The model under review builds one solid part; all positions refer to its coordinate system, in mm. A direction names the side the tool comes from. Give positions to 0.01 mm unless a question says otherwise; leave off trailing zeros. Write each loop counter-clockwise with the first axis right and the second up, starting at its lowest first coordinate (ties: lowest second). Pieces come first, ordered by that corner, then holes. Notation, with made-up numbers: (52.5, -27) -> (105.5, -27) arc R23 cw to (105.5, -19) -> close; hole circle Ø5 at (56.25, 46). An arc over 180 degrees is marked (long way). Use CSV: the item, a comma, the result in double quotes.
```python
from build123d import *

# Parameters (mm, degrees)
F1_DEPTH = 30
F2_R     = 0.5


with BuildPart() as f1:
    # F0 (on Front) → F1 (new body, symmetric)
    with BuildSketch(Plane.XZ):
        Polygon((-63.04628, 0), (0, 0), (0, 3), (-4.215537, 9.893654), (-3, 3), (-15, 3), (-22.38508, 44.88287), (-25.860448, 47.316349), (-18.04628, 3), (-63.04628, 3), align=None)
    extrude(amount=F1_DEPTH, both=True)

    # F2
    f2_edges = [f1.edges().sort_by_distance(p)[0] for p in [
        (-22.38508, 0, 44.88287),
        (-4.215537, 0, 9.893654),
        (-25.860448, 0, 47.316349),
    ]]
    fillet(f2_edges, radius=F2_R)


solid = f1.part
```
Q1. Consider section C-C (x = -19.5). Write out the cut boundary in (y, z).
Derived:
outline,"(-30, 0) -> (30, 0) -> (30, 3) -> (-30, 3) -> close; (-30, 11.24) -> (30, 11.24) -> (30, 28.52) -> (-30, 28.52) -> close"
Q2. Insertion check: pin 1 (22.5 mm diameter, centred on x = -45, y = 6.5, fed in from +Z); pin 2 (13 mm diameter, centred on x = -8.5, y = -9.5, fed in from +Z). Each pin has a flat end and moves straight along its axis. Give the tip position at first contact, or say it passes through.
Derived:
pin 1,"stops at z = 3"
pin 2,"stops at z = 7.88"
Q3. The part is to be moulded in two halves that separate along X. For faces 4 (the flat face through (-9, 0, 3)), 5 (the flat face through (-27, 30, 2.7)), 6 (the flat face through (-21.902, -0.42, 24.866)), say which applies: pulls with the +X half, pulls with the -X half, needs draft (parallel to the pull), parting line crosses it, or undercut.
Derived:
face 4,"undercut"
face 5,"needs draft"
face 6,"pulls with the -X half"
Q4. Machinability: for faces 1 (the flat face through (-32, 0, 0)), 2 (the flat face through (-40, 0, 3)), 3 (the flat face through (-3.384, -0.42, 5.177)), which of the approach directions +Z, -Z, +X, -X, +Y, -Y give a long, thin tool a straight path to every point of the face, cutting with its end or side? Answer none if there is none.
Derived:
face 1,"-Z, +X, -X, +Y, -Y"
face 2,"-X, +Y, -Y"
face 3,"+Y, -Y"
Q5. To check wall thickness, follow probe 1 along Z at (x, y) = (-56, -17); probe 2 along X at (y, z) = (27.5, 4); probe 3 along X at (y, z) = (-9, 8). State the ranges of each line that lie inside material, in increasing order.
Derived:
probe 1,"z = 0 to 3"
probe 2,"x = -18.22 to -15.18, -3.18 to -0.61"
probe 3,"x = -18.93 to -15.88"
Q6. Consider section D-D (x = -10). Write out the cut boundary in (y, z), then the cut area to 3 significant figures.
Derived:
outline,"(-30, 0) -> (30, 0) -> (30, 3) -> (-30, 3) -> close"
area,"180 mm2"
Q7. Consider section B-B (z = 5). Write out the cut boundary in (x, y), then the cut area to 3 significant figures.
Derived:
outline,"(-18.4, -30) -> (-15.35, -30) -> (-15.35, 30) -> (-18.4, 30) -> close; (-3.35, -30) -> (-1.22, -30) -> (-1.22, 30) -> (-3.35, 30) -> close"
area,"311 mm2"
Q8. Consider section A-A (y = 9). Write out the cut boundary in (x, z).
Derived:
outline,"(-63.05, 0) -> (0, 0) -> (0, 3) -> (-2.84, 7.64) arc R0.5 ccw to (-3.76, 7.29) -> (-3, 3) -> (-15, 3) -> (-22.35, 44.68) arc R0.5 ccw to (-22.55, 45) -> (-24.87, 46.62) arc R0.5 ccw to (-25.65, 46.13) -> (-18.05, 3) -> (-63.05, 3) -> close"
